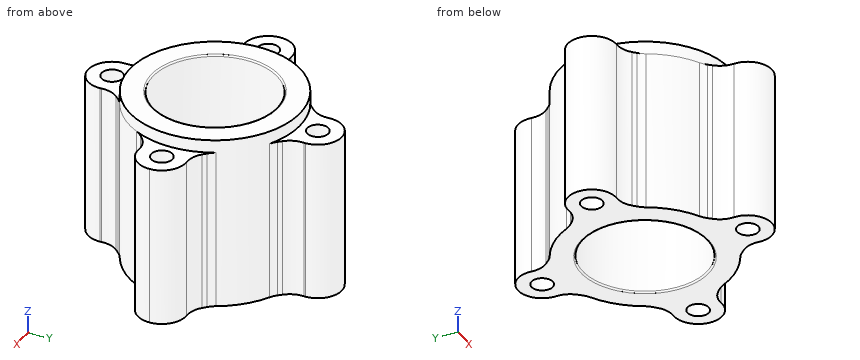
```python
from build123d import *

# Parameters (mm, degrees)
F0_R     = 3.3655
F0_R_2   = 20.32
F1_DEPTH = 50.8
F2_R     = 7.62
F3_R     = 26.9875
F3_R_2   = 19.685
F4_DEPTH = 54.864
F5_R     = 0.508


with BuildPart() as f1:
    # F0 (on Top) → F1 (new body)
    with BuildSketch(Plane.XY):
        with BuildLine():
            ThreePointArc((-11.5499308761, 24.3910691239), (-8.0975226707, 25.7440339273), (-4.4922459427, 26.6109917636))
            ThreePointArc((-4.4922459427, 26.6109917636), (-5.8575862517, 27.8922864976), (-6.8692513658, 29.4678511747))
            Line((-6.8692513658, 29.4678511747), (-11.5499308761, 24.3910691239))
        make_face()
        with BuildLine():
            ThreePointArc((4.4922459427, 26.6109917636), (8.0975226707, 25.7440339273), (11.5499308761, 24.3910691239))
            Line((11.5499308761, 24.3910691239), (6.8692513658, 29.4678511747))
            ThreePointArc((6.8692513658, 29.4678511747), (5.8575862517, 27.8922864976), (4.4922459427, 26.6109917636))
        make_face()
        with BuildLine():
            ThreePointArc((-4.4922459427, 26.6109917636), (0, 26.9875), (4.4922459427, 26.6109917636))
            ThreePointArc((4.4922459427, 26.6109917636), (5.8575862517, 27.8922864976), (6.8692513658, 29.4678511747))
            ThreePointArc((6.8692513658, 29.4678511747), (7.4299426447, 31.0747423921), (7.62, 32.766))
            ThreePointArc((7.62, 32.766), (-1.6912576079, 40.1959426447), (-6.8692513658, 29.4678511747))
            ThreePointArc((-6.8692513658, 29.4678511747), (-5.8575862517, 27.8922864976), (-4.4922459427, 26.6109917636))
        make_face()
        with Locations((0, 32.766)):
            Circle(F0_R, mode=Mode.SUBTRACT)
        with BuildLine():
            ThreePointArc((-4.4922459427, 26.6109917636), (0, 25.146), (4.4922459427, 26.6109917636))
            ThreePointArc((4.4922459427, 26.6109917636), (0, 26.9875), (-4.4922459427, 26.6109917636))
        make_face()
        with BuildLine():
            ThreePointArc((-26.6109917636, 4.4922459427), (-25.7440339273, 8.0975226707), (-24.3910691239, 11.5499308761))
            Line((-24.3910691239, 11.5499308761), (-29.4678511747, 6.8692513658))
            ThreePointArc((-29.4678511747, 6.8692513658), (-27.8922864976, 5.8575862517), (-26.6109917636, 4.4922459427))
        make_face()
        with BuildLine():
            ThreePointArc((-26.6109917636, -4.4922459427), (-26.9875, 0), (-26.6109917636, 4.4922459427))
            ThreePointArc((-26.6109917636, 4.4922459427), (-27.8922864976, 5.8575862517), (-29.4678511747, 6.8692513658))
            ThreePointArc((-29.4678511747, 6.8692513658), (-40.386, 0), (-29.4678511747, -6.8692513658))
            ThreePointArc((-29.4678511747, -6.8692513658), (-27.8922864976, -5.8575862517), (-26.6109917636, -4.4922459427))
        make_face()
        with Locations((-32.766, 0)):
            Circle(F0_R, mode=Mode.SUBTRACT)
        with BuildLine():
            ThreePointArc((-25.146, 0), (-25.521499922, 2.3625449454), (-26.6109917636, 4.4922459427))
            ThreePointArc((-26.6109917636, 4.4922459427), (-26.9875, 0), (-26.6109917636, -4.4922459427))
            ThreePointArc((-26.6109917636, -4.4922459427), (-25.521499922, -2.3625449454), (-25.146, 0))
        make_face()
        with BuildLine():
            ThreePointArc((-24.3910691239, -11.5499308761), (-25.7440339273, -8.0975226707), (-26.6109917636, -4.4922459427))
            ThreePointArc((-26.6109917636, -4.4922459427), (-27.8922864976, -5.8575862517), (-29.4678511747, -6.8692513658))
            Line((-29.4678511747, -6.8692513658), (-24.3910691239, -11.5499308761))
        make_face()
        with BuildLine():
            ThreePointArc((-6.8692513658, -29.4678511747), (-5.8575862517, -27.8922864976), (-4.4922459427, -26.6109917636))
            ThreePointArc((-4.4922459427, -26.6109917636), (-8.0975226707, -25.7440339273), (-11.5499308761, -24.3910691239))
            Line((-11.5499308761, -24.3910691239), (-6.8692513658, -29.4678511747))
        make_face()
        with BuildLine():
            ThreePointArc((-4.4922459427, -26.6109917636), (0, -26.9875), (4.4922459427, -26.6109917636))
            ThreePointArc((4.4922459427, -26.6109917636), (0, -25.146), (-4.4922459427, -26.6109917636))
        make_face()
        with BuildLine():
            ThreePointArc((6.8692513658, -29.4678511747), (5.8575862517, -27.8922864976), (4.4922459427, -26.6109917636))
            ThreePointArc((4.4922459427, -26.6109917636), (0, -26.9875), (-4.4922459427, -26.6109917636))
            ThreePointArc((-4.4922459427, -26.6109917636), (-5.8575862517, -27.8922864976), (-6.8692513658, -29.4678511747))
            ThreePointArc((-6.8692513658, -29.4678511747), (-1.6912576079, -40.1959426447), (7.62, -32.766))
            ThreePointArc((7.62, -32.766), (7.4299426447, -31.0747423921), (6.8692513658, -29.4678511747))
        make_face()
        with Locations((0, -32.766)):
            Circle(F0_R, mode=Mode.SUBTRACT)
        with BuildLine():
            Line((6.8692513658, -29.4678511747), (11.5499308761, -24.3910691239))
            ThreePointArc((11.5499308761, -24.3910691239), (8.0975226707, -25.7440339273), (4.4922459427, -26.6109917636))
            ThreePointArc((4.4922459427, -26.6109917636), (5.8575862517, -27.8922864976), (6.8692513658, -29.4678511747))
        make_face()
        with BuildLine():
            ThreePointArc((29.4678511747, -6.8692513658), (27.8922864976, -5.8575862517), (26.6109917636, -4.4922459427))
            ThreePointArc((26.6109917636, -4.4922459427), (25.7440339273, -8.0975226707), (24.3910691239, -11.5499308761))
            Line((24.3910691239, -11.5499308761), (29.4678511747, -6.8692513658))
        make_face()
        with BuildLine():
            ThreePointArc((29.4678511747, 6.8692513658), (27.8922864976, 5.8575862517), (26.6109917636, 4.4922459427))
            ThreePointArc((26.6109917636, 4.4922459427), (26.8932082176, 2.2539982288), (26.9875, 0))
            ThreePointArc((26.9875, 0), (26.8932082176, -2.2539982288), (26.6109917636, -4.4922459427))
            ThreePointArc((26.6109917636, -4.4922459427), (27.8922864976, -5.8575862517), (29.4678511747, -6.8692513658))
            ThreePointArc((29.4678511747, -6.8692513658), (36.8238631046, -6.4496625512), (40.386, 0))
            ThreePointArc((40.386, 0), (36.8238631046, 6.4496625512), (29.4678511747, 6.8692513658))
        make_face()
        with Locations((32.766, 0)):
            Circle(F0_R, mode=Mode.SUBTRACT)
        with BuildLine():
            ThreePointArc((26.9875, 0), (26.8932082176, 2.2539982288), (26.6109917636, 4.4922459427))
            ThreePointArc((26.6109917636, 4.4922459427), (25.146, 0), (26.6109917636, -4.4922459427))
            ThreePointArc((26.6109917636, -4.4922459427), (26.8932082176, -2.2539982288), (26.9875, 0))
        make_face()
        with BuildLine():
            Line((29.4678511747, 6.8692513658), (24.3910691239, 11.5499308761))
            ThreePointArc((24.3910691239, 11.5499308761), (25.7440339273, 8.0975226707), (26.6109917636, 4.4922459427))
            ThreePointArc((26.6109917636, 4.4922459427), (27.8922864976, 5.8575862517), (29.4678511747, 6.8692513658))
        make_face()
        with BuildLine():
            ThreePointArc((26.6109917636, 4.4922459427), (25.7440339273, 8.0975226707), (24.3910691239, 11.5499308761))
            ThreePointArc((24.3910691239, 11.5499308761), (19.0830442573, 19.0830442573), (11.5499308761, 24.3910691239))
            ThreePointArc((11.5499308761, 24.3910691239), (8.0975226707, 25.7440339273), (4.4922459427, 26.6109917636))
            ThreePointArc((4.4922459427, 26.6109917636), (0, 25.146), (-4.4922459427, 26.6109917636))
            ThreePointArc((-4.4922459427, 26.6109917636), (-8.0975226707, 25.7440339273), (-11.5499308761, 24.3910691239))
            ThreePointArc((-11.5499308761, 24.3910691239), (-19.0830442573, 19.0830442573), (-24.3910691239, 11.5499308761))
            ThreePointArc((-24.3910691239, 11.5499308761), (-25.7440339273, 8.0975226707), (-26.6109917636, 4.4922459427))
            ThreePointArc((-26.6109917636, 4.4922459427), (-25.521499922, 2.3625449454), (-25.146, 0))
            ThreePointArc((-25.146, 0), (-25.521499922, -2.3625449454), (-26.6109917636, -4.4922459427))
            ThreePointArc((-26.6109917636, -4.4922459427), (-25.7440339273, -8.0975226707), (-24.3910691239, -11.5499308761))
            ThreePointArc((-24.3910691239, -11.5499308761), (-19.0830442573, -19.0830442573), (-11.5499308761, -24.3910691239))
            ThreePointArc((-11.5499308761, -24.3910691239), (-8.0975226707, -25.7440339273), (-4.4922459427, -26.6109917636))
            ThreePointArc((-4.4922459427, -26.6109917636), (0, -25.146), (4.4922459427, -26.6109917636))
            ThreePointArc((4.4922459427, -26.6109917636), (8.0975226707, -25.7440339273), (11.5499308761, -24.3910691239))
            ThreePointArc((11.5499308761, -24.3910691239), (19.0830442573, -19.0830442573), (24.3910691239, -11.5499308761))
            ThreePointArc((24.3910691239, -11.5499308761), (25.7440339273, -8.0975226707), (26.6109917636, -4.4922459427))
            ThreePointArc((26.6109917636, -4.4922459427), (25.146, 0), (26.6109917636, 4.4922459427))
        make_face()
        Circle(F0_R_2, mode=Mode.SUBTRACT)
        with BuildLine():
            ThreePointArc((-4.4922459427, 26.6109917636), (0, 26.9875), (4.4922459427, 26.6109917636))
            ThreePointArc((4.4922459427, 26.6109917636), (5.8575862517, 27.8922864976), (6.8692513658, 29.4678511747))
            ThreePointArc((6.8692513658, 29.4678511747), (7.4299426447, 31.0747423921), (7.62, 32.766))
            ThreePointArc((7.62, 32.766), (-1.6912576079, 40.1959426447), (-6.8692513658, 29.4678511747))
            ThreePointArc((-6.8692513658, 29.4678511747), (-5.8575862517, 27.8922864976), (-4.4922459427, 26.6109917636))
        make_face()
        with Locations((0, 32.766)):
            Circle(F0_R, mode=Mode.SUBTRACT)
        with BuildLine():
            ThreePointArc((-26.6109917636, -4.4922459427), (-26.9875, 0), (-26.6109917636, 4.4922459427))
            ThreePointArc((-26.6109917636, 4.4922459427), (-27.8922864976, 5.8575862517), (-29.4678511747, 6.8692513658))
            ThreePointArc((-29.4678511747, 6.8692513658), (-40.386, 0), (-29.4678511747, -6.8692513658))
            ThreePointArc((-29.4678511747, -6.8692513658), (-27.8922864976, -5.8575862517), (-26.6109917636, -4.4922459427))
        make_face()
        with Locations((-32.766, 0)):
            Circle(F0_R, mode=Mode.SUBTRACT)
        with BuildLine():
            ThreePointArc((29.4678511747, 6.8692513658), (27.8922864976, 5.8575862517), (26.6109917636, 4.4922459427))
            ThreePointArc((26.6109917636, 4.4922459427), (26.8932082176, 2.2539982288), (26.9875, 0))
            ThreePointArc((26.9875, 0), (26.8932082176, -2.2539982288), (26.6109917636, -4.4922459427))
            ThreePointArc((26.6109917636, -4.4922459427), (27.8922864976, -5.8575862517), (29.4678511747, -6.8692513658))
            ThreePointArc((29.4678511747, -6.8692513658), (36.8238631046, -6.4496625512), (40.386, 0))
            ThreePointArc((40.386, 0), (36.8238631046, 6.4496625512), (29.4678511747, 6.8692513658))
        make_face()
        with Locations((32.766, 0)):
            Circle(F0_R, mode=Mode.SUBTRACT)
        with BuildLine():
            ThreePointArc((6.8692513658, -29.4678511747), (5.8575862517, -27.8922864976), (4.4922459427, -26.6109917636))
            ThreePointArc((4.4922459427, -26.6109917636), (0, -26.9875), (-4.4922459427, -26.6109917636))
            ThreePointArc((-4.4922459427, -26.6109917636), (-5.8575862517, -27.8922864976), (-6.8692513658, -29.4678511747))
            ThreePointArc((-6.8692513658, -29.4678511747), (-1.6912576079, -40.1959426447), (7.62, -32.766))
            ThreePointArc((7.62, -32.766), (7.4299426447, -31.0747423921), (6.8692513658, -29.4678511747))
        make_face()
        with Locations((0, -32.766)):
            Circle(F0_R, mode=Mode.SUBTRACT)
    extrude(amount=F1_DEPTH)

    # F2
    f2_edges = [f1.edges().sort_by_distance(p)[0] for p in [
        (-6.869251, 29.467851, 25.4),
        (-29.467851, 6.869251, 25.4),
        (-29.467851, -6.869251, 25.4),
        (-24.391069, -11.549931, 25.4),
        (-11.549931, -24.391069, 25.4),
        (-6.869251, -29.467851, 25.4),
        (6.869251, -29.467851, 25.4),
        (11.549931, -24.391069, 25.4),
        (24.391069, -11.549931, 25.4),
        (29.467851, -6.869251, 25.4),
        (29.467851, 6.869251, 25.4),
        (24.391069, 11.549931, 25.4),
        (11.549931, 24.391069, 25.4),
        (6.869251, 29.467851, 25.4),
        (-11.549931, 24.391069, 25.4),
        (-24.391069, 11.549931, 25.4),
    ]]
    fillet(f2_edges, radius=F2_R)

    # F3 (on Top) → F4 (join)
    with BuildSketch(Plane.XY):
        Circle(F3_R)
        Circle(F3_R_2, mode=Mode.SUBTRACT)
    extrude(amount=F4_DEPTH)

    # F5
    f5_edges = [f1.edges().sort_by_distance(p)[0] for p in [
        (-19.685, 0, 54.864),
        (-19.685, 0, 0),
    ]]
    fillet(f5_edges, radius=F5_R)


solid = f1.part
```
Here's how the part is built. I have some questions about the finished solid (model axes, mm). Give positions to 0.01 mm unless a question says otherwise; leave off trailing zeros. Order: outer loops, then holes, each group sorted by start corner. A loop starts at its lowest first (then second) coordinate and runs counter-clockwise, first axis right, second up. Notation, with made-up numbers: M 10.25,-26 L 48.25,-26 A14 ccw 48.25,-11 Z; hole C 83.5,84 d5. An arc over 180 degrees is marked long. Use a Markdown table: item, result. Add a question column.
1. For pin 1 Ø1 at (y, z) = (-11, 36.5) entering from +X; pin 2 Ø5.5 at (x, y) = (0, 32.766) entering from +Z; pin 3 Ø13 at (x, y) = (-0.5, 36) entering from +Z; pin 4 Ø12 at (x, z) = (-20, 31) entering from +Y, each with a flat end and sliding along its axis, tell me the tip position at first contact or that it passes through.
2. Suppose I cut it at A-A (x = 0). List the corners of the cut face in (y, z) for me (1 decimal), and give its area (3 significant figures).
3. Suppose I cut it at C-C (x = -22.5). List the corners of the cut face in (y, z) for me.
4. I need wall thicknesses on probe 1 along Y at (x, z) = (0, 37) (1 decimal); probe 2 along Y at (x, z) = (-33, 16.5); probe 3 along Y at (x, z) = (6.5, 30.5). Which ranges of each line are inside material? Lowest first, please. Write a range as from..to.
5. Suppose I cut it at B-B (z = 40.5). Give the number of separate pieces and of enclosed holes in the cut face, and give its area (3 significant figures).
Results list:
| question | item | result |
|---|---|---|
| 1 | pin 1 | stops at x = 25.53 |
| 1 | pin 2 | passes through |
| 1 | pin 3 | stops at z = 50.8 |
| 1 | pin 4 | stops at y = 23.07 |
| 2 | outline | M -40.4,0 L -36.1,0 L -36.1,50.8 L -40.4,50.8 Z; M -29.4,0 L -20.2,0 A0.5 ccw -19.7,0.5 L -19.7,54.4 A0.5 ccw -20.2,54.9 L -27,54.9 L -27,50.8 L -29.4,50.8 Z; M 19.7,0.5 A0.5 ccw 20.2,0 L 29.4,0 L 29.4,50.8 L 27,50.8 L 27,54.9 L 20.2,54.9 A0.5 ccw 19.7,54.4 Z; M 36.1,0 L 40.4,0 L 40.4,50.8 L 36.1,50.8 Z |
| 2 | area | 1,480 mm² |
| 3 | outline | M -14.9,0 L 14.9,0 L 14.9,54.86 L -14.9,54.86 Z |
| 4 | probe 1 | y = -40.4..-36.1, -29.4..-19.7, 19.7..29.4, 36.1..40.4 |
| 4 | probe 2 | y = -7.62..-3.36, 3.36..7.62 |
| 4 | probe 3 | y = -36.74..-18.58, 18.58..36.74 |
| 5 | separate pieces | 1 |
| 5 | enclosed holes | 5 |
| 5 | area | 1,720 mm² |
